```python
from build123d import *

# Parameters (mm, degrees)
SKETCH1_W           = 1370
SKETCH1_H           = 900
BOSS_EXTRUDE1_DEPTH = 6.35
CUT_EXTRUDE1_REACH  = 1641.189
SKETCH2_W           = 1050
SKETCH2_H           = 300


with BuildPart() as part:
    # Sketch1 → Boss-Extrude1 (new body)
    with BuildSketch(Plane(origin=(0, 0, 0), x_dir=(1, 0, 0), z_dir=(0, 1, 0))):
        with Locations((685, 450)):
            Rectangle(SKETCH1_W, SKETCH1_H)
    extrude(amount=BOSS_EXTRUDE1_DEPTH)

    # Sketch2 → Cut-Extrude1 (cut, up to next)
    with BuildSketch(Plane(origin=(0, 6.35, 0), x_dir=(1, 0, 0), z_dir=(0, 1, 0)), mode=Mode.PRIVATE) as cut_extrude1_sk1:
        with Locations((685, 245)):
            Rectangle(SKETCH2_W, SKETCH2_H)
    cut_extrude1_tool1 = extrude(cut_extrude1_sk1.sketch, amount=-CUT_EXTRUDE1_REACH, mode=Mode.PRIVATE) & part.part
    add(cut_extrude1_tool1.solids().sort_by_distance((685, 6.35, -245))[0], mode=Mode.SUBTRACT)


solid = part.part
```
The listing builds one solid part. Answer for the finished solid, in the listing's coordinates (mm). Give positions to 0.01 mm unless a question says otherwise; leave off trailing zeros. Loops run counter-clockwise (first coordinate to the right, second up) from the corner with the lowest first, then second, coordinate; pieces in that order, holes last. Notation, with made-up numbers: (-34, -9) - (-15, -9) arc R32 cw to (-15, 22) - close; hole circle Ø11 at (45, 53). An arc over 180 degrees is marked (long way). Return JSON: item names as keys, results as strings. Group by question number.
1. Find section B-B (z = -331.5). Write down the section's boundary in (x, y), then the cut area to 3 significant figures.
2. Find section A-A (x = 674). Write down the section's boundary in (y, z), then the cut area to 3 significant figures.
3. Given pin 1 Ø5 at (x, z) = (528, -743) entering from -Y, flat-ended and moving along its own axis, determine where the tip first touches the part or whether it passes through.
4. Find section C-C (y = 4.5). Write down the section's boundary in (x, z).
5. Straight lines are drawn through the part: line 1 (Z direction, x = 854.5, y = 5.75); line 2 (X direction, y = 1.5, z = -262). For each, find the intervals that lie inside material, in ascending order. Write a range as [from, to].
Verdict:
{
 "1": {"outline": "(0, 0) - (160, 0) - (160, 6.35) - (0, 6.35) - close; (1210, 0) - (1370, 0) - (1370, 6.35) - (1210, 6.35) - close", "area": "2,030 mm^2"},
 "2": {"outline": "(0, -900) - (6.35, -900) - (6.35, -395) - (0, -395) - close; (0, -95) - (6.35, -95) - (6.35, 0) - (0, 0) - close", "area": "3,810 mm^2"},
 "3": {"pin 1": "stops at y = 0"},
 "4": {"outline": "(0, -900) - (1370, -900) - (1370, 0) - (0, 0) - close; hole (160, -395) - (1210, -395) - (1210, -95) - (160, -95) - close"},
 "5": {"line 1": "z = [-900, -395], [-95, 0]", "line 2": "x = [0, 160], [1210, 1370]"}
}
